Here's the drawing with two shaded views (mm, measured from the low corner). I have some questions. Coordinates: 2 decimals unless noted, no trailing zeros. Order: outer loops, then holes, each group sorted by start corner. A loop starts at its lowest first (then second) coordinate and runs counter-clockwise, first axis right, second up. Notation, with made-up numbers: (29.25, 78.25) - (45.25, 78.25) arc R16 cw to (45.25, 98.25) - close; hole circle Ø4 at (-4.5, 72.25). An arc over 180 degrees is marked (long way). Answer as a JSON object with one key per item and string values. Group by question number.
(1) We'd pull the mould along Z, two halves only. Please class the marked faces 1, 2, 3 and 4: pulls with the +Z half, pulls with the -Z half, needs draft (parallel to the pull), parting line crosses it, or undercut.
(2) Will these pins go through, and if not, where does the flat tip stop? P1, Ø1, axis at y = 7.5, z = 73.5, coming from the +X side; P2, Ø2, axis at x = 16, y = 7, coming from the +Z side (1 decimal); P3, Ø5, axis at y = 6.5, z = 46, coming from the +X side.
(3) Imagine slicing it at C-C, the plane z = 60.5. Write out the boundary of the cut face in (x, y), and give its area (3 significant figures).
(4) Imagine slicing it at A-A, the plane y = 6.25. Write out the boundary of the cut face in (x, z).
(5) Imagine slicing it at B-B, the plane x = 57.5. Write out the boundary of the cut face in (y, z).
(6) Please list where these lines run through material, in increasing order: probe 1 along X at (y, z) = (5.75, 49.5); probe 2 along X at (y, z) = (8.5, 47) (1 decimal); probe 3 along Z at (x, y) = (71, 7) (1 decimal).
(7) Imagine slicing it at D-D, the plane x = 86.5. Write out the boundary of the cut face in (y, z).
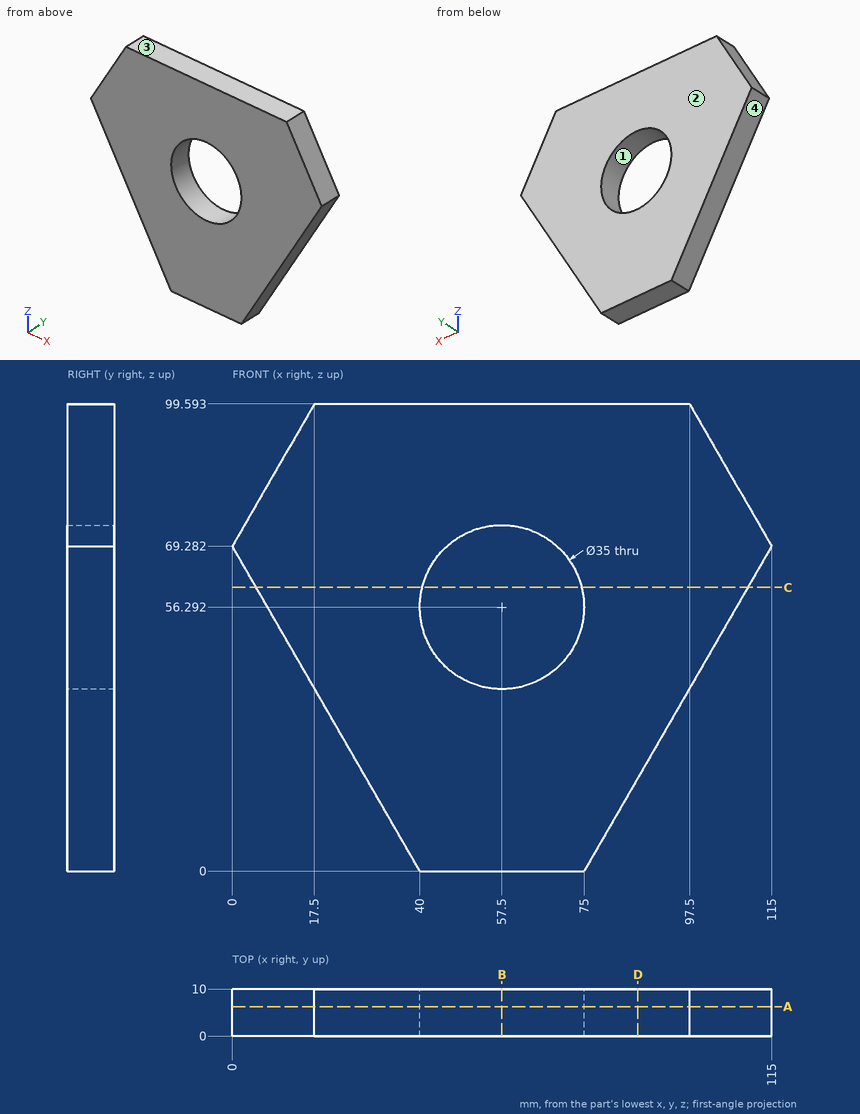
Result set:
{
 "1": {"face 1": "undercut", "face 2": "needs draft", "face 3": "pulls with the +Z half", "face 4": "pulls with the -Z half"},
 "2": {"P1": "stops at x = 112.85", "P2": "stops at z = 98.7", "P3": "stops at x = 103"},
 "3": {"outline": "(5.07, 0) - (40.51, 0) - (40.51, 10) - (5.07, 10) - close; (74.49, 0) - (109.93, 0) - (109.93, 10) - (74.49, 10) - close", "area": "709 mm^2"},
 "4": {"outline": "(0, 69.28) - (40, 0) - (75, 0) - (115, 69.28) - (97.5, 99.59) - (17.5, 99.59) - close; hole circle Ø35 at (57.5, 56.29)"},
 "5": {"outline": "(0, 0) - (10, 0) - (10, 38.79) - (0, 38.79) - close; (0, 73.79) - (10, 73.79) - (10, 99.59) - (0, 99.59) - close"},
 "6": {"probe 1": "x = 11.42 to 41.37, 73.63 to 103.58", "probe 2": "x = 12.9 to 42.7, 72.3 to 102.1", "probe 3": "z = 0 to 45.2, 67.4 to 99.6"},
 "7": {"outline": "(0, 19.92) - (10, 19.92) - (10, 99.59) - (0, 99.59) - close"}
}
